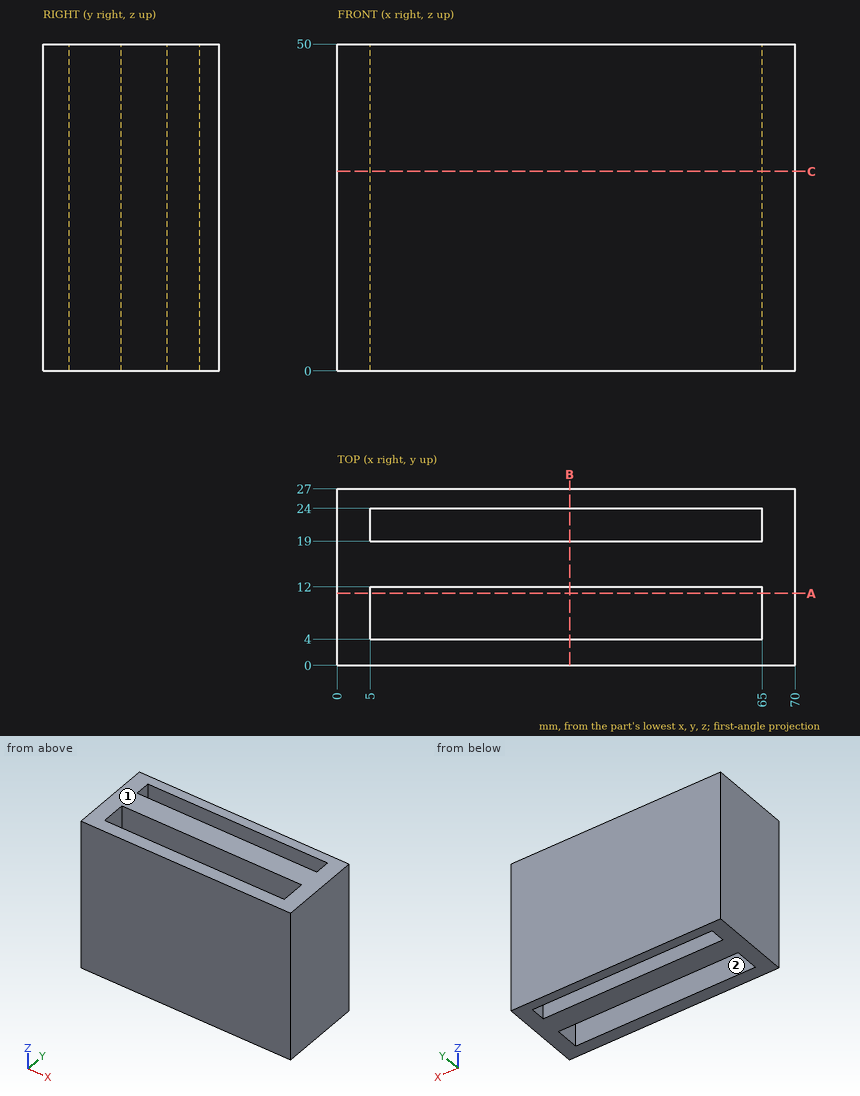
Source: three-view drawing plus pictorial views. Frame: mm from the lowest corner of the part. A direction names the side the tool comes from. Give positions to 0.01 mm unless a question says otherwise; leave off trailing zeros. Write each loop counter-clockwise with the first axis right and the second up, starting at its lowest first coordinate (ties: lowest second). Pieces come first, ordered by that corner, then holes. Notation, with made-up numbers: (75.5, -37.5) - (132.5, -37.5) arc R11 ccw to (132.5, -17.5) - close; hole circle Ø11 at (20.25, 56.25). An arc over 180 degrees is marked (long way). Write item = value, one per line. Start each with the question number.
1. Ray query, L1, parallel to Y at x = 39, z = 35; L2, parallel to X at y = 8.5, z = 40.5. Return the intervals inside material, ascending.
2. Section query C-C, the plane z = 30.5. Output: boundary loops of the cut face in (x, y), then the cut area to 3 significant figures.
3. Section query A-A, the plane y = 11. Output: boundary loops of the cut face in (x, z).
4. Section query B-B, the plane x = 35.5. Output: boundary loops of the cut face in (y, z).
5. Access query for the marked faces 1 and 2. Directions: +Z, -Z, +X, -X, +Y, -Y. A direction counts if a zero-diameter tool reaches every point of the face in a straight line with its end or side. Return the directions, or none.
Check sheet entries:
q1.L1 = 0 to 4, 12 to 19, 24 to 27
q1.L2 = 0 to 5, 65 to 70
q2.outline = (0, 0) - (70, 0) - (70, 27) - (0, 27) - close; hole (5, 4) - (65, 4) - (65, 12) - (5, 12) - close; hole (5, 19) - (65, 19) - (65, 24) - (5, 24) - close
q2.area = 1,110 mm2
q3.outline = (0, 0) - (5, 0) - (5, 50) - (0, 50) - close; (65, 0) - (70, 0) - (70, 50) - (65, 50) - close
q4.outline = (0, 0) - (4, 0) - (4, 50) - (0, 50) - close; (12, 0) - (19, 0) - (19, 50) - (12, 50) - close; (24, 0) - (27, 0) - (27, 50) - (24, 50) - close
q5.face_1 = +Z, +X, -X, +Y, -Y
q5.face_2 = +Z, -Z
